Autodesk Fusion 360 part; units mm, degrees
sketch "スケッチ1" plane through (0, 0, 0) normal (1, 0, 0) x (0, 0, -1)
  line L0 (-116, 0) -> (-116, 20)
  line L1 (-116, 20) -> (-111.3943, 33.2207)
  line L2 (-111.3943, 33.2207) -> (-101.951, 29.931)
  line L3 (-101.951, 29.931) -> (-105.2407, 20.4876)
  line L4 (-105.2407, 20.4876) -> (-95.7973, 17.1978)
  line L5 (-14, 252) -> (0, 252)
  line L6 (-95.7973, 17.1978) -> (-79.3485, 64.4147)
  line L7 (-79.3485, 64.4147) -> (-65.1834, 59.4801)
  line L8 (-65.1834, 59.4801) -> (-63.8675, 63.2574)
  line L9 (-63.8675, 63.2574) -> (-78.0326, 68.1921)
  line L10 (-78.0326, 68.1921) -> (-38.5555, 181.5127)
  line L11 (-38.5555, 181.5127) -> (-24.3904, 176.578)
  line L12 (-24.3904, 176.578) -> (-23.0745, 180.3554)
  line L13 (-23.0745, 180.3554) -> (-37.2396, 185.29)
  line L14 (-37.2396, 185.29) -> (-14, 252)
  line L15 (-116, 0) -> (-70, 0)
  line L16 (-70, 0) -> (-70, -4)
  line L17 (-70, -4) -> (-50, -4)
  line L18 (-50, -4) -> (-50, 0)
  line L19 (-50, 0) -> (0, 0)
  line L20 (0, 252) -> (0, 165)
  line L21 (0, 165) -> (4, 165)
  line L22 (4, 165) -> (4, 145)
  line L23 (4, 145) -> (0, 145)
  line L24 (0, 145) -> (0, 0)
  line L25 (4, 155) -> (-13.5, 155)
  line L26 (-60, -4) -> (-60, 13.5)
  line L27 (-64.1481, 77.6509) -> (-33.5533, 165.4743)
  line L28 (-10, 10) -> (-30, 10)
  line L29 (-30, 10) -> (-30, 30)
  line L30 (-30, 30) -> (-10, 30)
  line L31 (-10, 30) -> (-10, 10)
  line L32 (-108, 8) -> (-90, 8)
  line L33 (-102.8799, 19.6651) -> (-98.1582, 18.0203)
  line L34 (-98.1582, 18.0203) -> (-99.1451, 15.1873)
  line L35 (-99.1451, 15.1873) -> (-103.8668, 16.8321)
  line L36 (-103.8668, 16.8321) -> (-102.8799, 19.6651)
  dimension "d1" = 116
  dimension "d2" = 20
  dimension "d3" = 14
  dimension "d4" = 10
  dimension "d5" = 10
  dimension "d6" = 10
  dimension "d9" = 14
  dimension "d11" = 252
  dimension "d12" = 248.642
  dimension "d13" = 4
  dimension "d14" = 4
  dimension "d15" = 120
  dimension "d16" = 50
  dimension "d17" = 15
  dimension "d18" = 20
  dimension "d19" = 4
  dimension "d20" = 50
  dimension "d21" = 4
  dimension "d22" = 20
  dimension "d23" = 145
  dimension "d24" = 17.5
  dimension "d25" = 17.5
  dimension "d31" = 10
  dimension "d32" = 13.5
  dimension "d33" = 13.5
  dimension "d36" = 10
  dimension "d37" = 20
  dimension "d38" = 20
  dimension "d39" = 10
  dimension "d40" = 8
  dimension "d41" = 8
  dimension "d42" = 18
  dimension "d43" = 5
  dimension "d44" = 3
extrude "押し出し1" add sketch "スケッチ1" along normal blind 4 contours L0 L1 L2 L3 L4 L5 L6 L7 L8 L9 L10 L11 L12 L13 L14 L15 L16 L17 L18 L19 L20 L21 L22 L23 L24 L34 L35 L36
hole "穴1" at (0, 155, 13.5) at (0, 13.5, 60) at (0, 77.6509, 64.1481) at (0, 165.4743, 33.5533) at (0, 8, 108) at (0, 8, 90) direction (1, 0, 0) diameter 3.2 end through all
fillet "フィレット1" radius 1 2 edges at (2, 29.931, 101.951) (2, 33.2207, 111.3943)
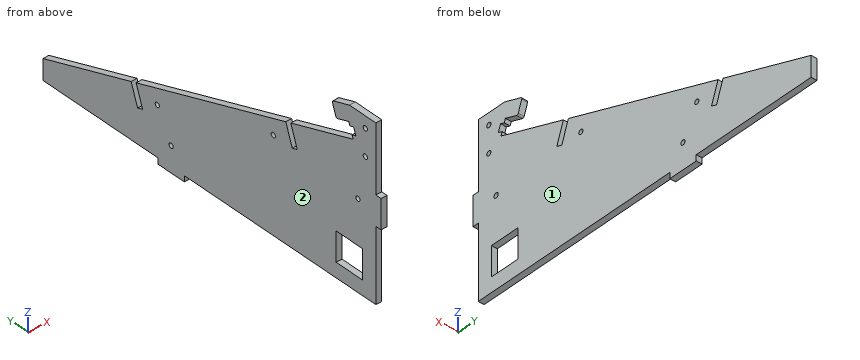
Work out the finished part from the listing and answer in its coordinate system (mm). Face numbers are marked on the shaded views. Give positions to 0.01 mm unless a question says otherwise; leave off trailing zeros. Loops run counter-clockwise (first coordinate to the right, second up) from the corner with the lowest first, then second, coordinate; pieces in that order, holes last. Notation, with made-up numbers: (49.25, 16) - (54.25, 16) arc R25 cw to (54.25, 31) - close; hole circle Ø6 at (68.25, -23.5). An arc over 180 degrees is marked (long way). Use CSV: the item, a comma, the result in double quotes. Start each with the question number.
(1) Find the intervals of material crossed by L1, parallel to Z at x = 1.65, y = 8; L2, parallel to Z at x = 3.25, y = 13.5; L3, parallel to Y at x = 3.15, z = 108, in increasing order.
(2) Find section A-A, the plane z = 6. Determine the outline of the cut face in (x, y), plus the area to 3 significant figures.
(3) Find section B-B, the plane y = 84.5. Determine the outline of the cut face in (x, z), plus the area to 3 significant figures.
(4) Determine the mould class of the marked faces 1 and 2 for opening direction X: released by +X, released by -X, zero draft, split by the parting line, or undercut.
(5) Each of these flat-tipped pins is pushed along its axis until it touches: pin 1 (2 mm diameter, centred on x = 2, y = 16, fed in from -Z); pin 2 (1.2 mm diameter, centred on x = 3, y = -1.5, fed in from +Z); pin 3 (1.5 mm diameter, centred on x = 1, z = 11, fed in from -Y). Where does it stop, or does it pass through?
(6) Find section C-C, the plane x = 1.1. Count the separate pieces of the cut face and the enclosed holes in it, plus the area to 3 significant figures.
Results found:
1,L1,"0 to 88.4, 91.6 to 106.4, 109.6 to 116"
1,L2,"0 to 10, 30 to 58.4, 61.6 to 116"
1,L3,"0 to 6.4, 9.6 to 32.04"
2,outline,"(0, 0) - (4, 0) - (4, 252) - (0, 252) - close"
2,area,"1,010 mm^2"
3,outline,"(0, 0) - (4, 0) - (4, 72.35) - (0, 72.35) - close"
3,area,"289 mm^2"
4,face 1,"released by +X"
4,face 2,"released by -X"
5,pin 1,"z = 0"
5,pin 2,"z = 70"
5,pin 3,"y = 0"
6,separate pieces,"1"
6,enclosed holes,"7"
6,area,"14,600 mm^2"
